```python
from build123d import *

# Parameters (mm, degrees)
SKETCH1_W           = 200
SKETCH1_H           = 200
BOSS_EXTRUDE1_DEPTH = 300
FILLET1_R           = 10
SHELL1_T            = -8
CUT_EXTRUDE1_DEPTH  = 44
FILLET2_R           = 25
FILLET3_R           = 25
CUT_EXTRUDE2_DEPTH  = 5.5


with BuildPart() as part:
    # Sketch1 → Boss-Extrude1 (new body)
    with BuildSketch(Plane(origin=(0, 0, 0), x_dir=(1, 0, 0), z_dir=(0, 1, 0))):
        Rectangle(SKETCH1_W, SKETCH1_H)
    extrude(amount=BOSS_EXTRUDE1_DEPTH)

    # Fillet1
    fillet1_edges = [part.edges().sort_by_distance(p)[0] for p in [
        (0, 0, -100),
        (100, 0, 0),
        (0, 0, 100),
        (-100, 0, 0),
        (-100, 150, -100),
        (100, 150, -100),
        (100, 150, 100),
        (-100, 150, 100),
    ]]
    fillet(fillet1_edges, radius=FILLET1_R)

    # Shell1
    shell1_openings = [part.faces().sort_by_distance(p)[0] for p in [
        (0, 300, 0),
    ]]
    offset(amount=SHELL1_T, openings=shell1_openings, kind=Kind.INTERSECTION)

    # Sketch2 → Cut-Extrude1 (cut)
    with BuildSketch(Plane(origin=(0, 0, -100), x_dir=(-1, 0, 0), z_dir=(0, 0, -1))):
        with BuildLine():
            Line((62, 100), (-28, 100))
            Line((-28, 100), (-28, 130))
            ThreePointArc((-28, 130), (-57.029416855, 206), (-28, 282))
            Line((-28, 282), (-28, 300))
            Line((-28, 300), (62, 300))
            Line((62, 300), (62, 100))
        make_face()
    extrude(amount=-CUT_EXTRUDE1_DEPTH, mode=Mode.SUBTRACT)

    # Fillet2
    fillet2_edges = [part.edges().sort_by_distance(p)[0] for p in [
        (28, 130, -96),
    ]]
    fillet(fillet2_edges, radius=FILLET2_R)

    # Fillet3
    fillet3_edges = [part.edges().sort_by_distance(p)[0] for p in [
        (28, 282, -96),
    ]]
    fillet(fillet3_edges, radius=FILLET3_R)

    # Sketch3 → Cut-Extrude2 (cut)
    with BuildSketch(Plane(origin=(0, 300, 0), x_dir=(1, 0, 0), z_dir=(0, 1, 0))):
        with BuildLine():
            Line((28, 92), (90, 92))
            ThreePointArc((90, 92), (91.414213562, 91.414213562), (92, 90))
            Line((92, 90), (92, -90))
            ThreePointArc((92, -90), (91.414213562, -91.414213562), (90, -92))
            Line((90, -92), (-90, -92))
            ThreePointArc((-90, -92), (-91.414213562, -91.414213562), (-92, -90))
            Line((-92, -90), (-92, 90))
            ThreePointArc((-92, 90), (-91.414213562, 91.414213562), (-90, 92))
            Line((-90, 92), (-62, 92))
            Line((-62, 92), (-62, 94.5))
            Line((-62, 94.5), (-90, 94.5))
            ThreePointArc((-90, 94.5), (-93.181980515, 93.181980515), (-94.5, 90))
            Line((-94.5, 90), (-94.5, -90))
            ThreePointArc((-94.5, -90), (-93.181980515, -93.181980515), (-90, -94.5))
            Line((-90, -94.5), (90, -94.5))
            ThreePointArc((90, -94.5), (93.181980515, -93.181980515), (94.5, -90))
            Line((94.5, -90), (94.5, 90))
            ThreePointArc((94.5, 90), (93.181980515, 93.181980515), (90, 94.5))
            Line((90, 94.5), (28, 94.5))
            Line((28, 94.5), (28, 92))
        make_face()
    extrude(amount=-CUT_EXTRUDE2_DEPTH, mode=Mode.SUBTRACT)


solid = part.part
```
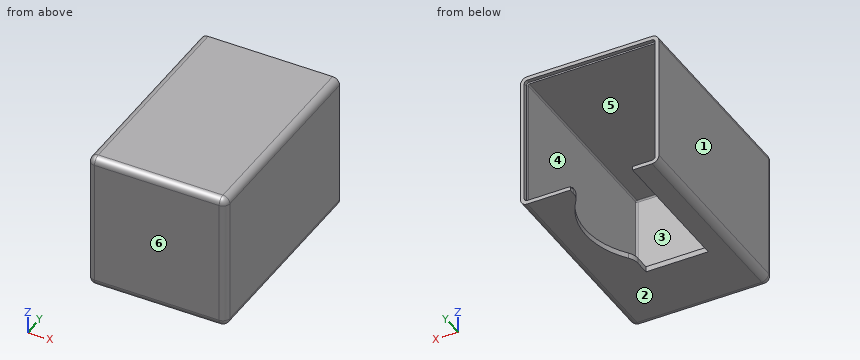
Geometry: final body of the model. Coordinates: model frame, mm. Face numbers are marked on the shaded views. A direction names the side the tool comes from. Coordinates: 2 decimals unless noted, no trailing zeros. Order: outer loops, then holes, each group sorted by start corner. A loop starts at its lowest first (then second) coordinate and runs counter-clockwise, first axis right, second up. Notation, with made-up numbers: (67, -1.5) - (110, -1.5) arc R19 ccw to (110, 22.5) - close; hole circle Ø10 at (-12, -36). An arc over 180 degrees is marked (long way). Return JSON: item names as keys, results as strings. Group by question number.
1. Cut plane B-B (x = -84). Output: boundary loops of the cut face in (y, z).
2. Pin query (flat end, axial travel): pin 1 (4 mm diameter, centred on y = 108.5, z = -94.5, fed in from -X); pin 2 (6 mm diameter, centred on x = -50.5, z = 62.5, fed in from +Y); pin 3 (4 mm diameter, centred on y = 295.5, z = -97, fed in from -X). Return the tip coordinate at first contact, or that it passes through.
3. Cut plane C-C (y = 71). Output: boundary loops of the cut face in (x, z).
4. Cut plane D-D (z = 46). Output: boundary loops of the cut face in (x, y).
5. Cut plane A-A (y = 104). Output: boundary loops of the cut face in (x, z), plus the area to 3 significant figures.
6. Set-up query: the marked faces 5 and 6. Return all of +Z, -Z, +X, -X, +Y, -Y with unobstructed straight access to the full face (end or side cutting, diameter ignored); none if empty.
7. Material intervals for line 1 along Z through (x, y) = (65.5, 110.5); line 2 along Y through (x, z) = (47, 18), sorted ascending. Write a range as [from, to].
8. Pull-direction query (X, two-part tool) for the marked faces 1, 2, 3 and 4; classes: pulls with the +X half, pulls with the -X half, needs draft (parallel to the pull), parting line crosses it, or undercut.
Resolved:
{
 "1": {"outline": "(0, -90) arc R10 ccw to (10, -100) - (300, -100) - (300, -94.5) - (294.5, -94.5) - (294.5, -92) - (10, -92) arc R2 cw to (8, -90) - (8, 90) arc R2 cw to (10, 92) - (294.5, 92) - (294.5, 94.5) - (300, 94.5) - (300, 100) - (10, 100) arc R10 ccw to (0, 90) - close"},
 "2": {"pin 1": "stops at x = -99.68", "pin 2": "stops at y = 8", "pin 3": "stops at x = -98.66"},
 "3": {"outline": "(-100, -90) arc R10 ccw to (-90, -100) - (90, -100) arc R10 ccw to (100, -90) - (100, 90) arc R10 ccw to (90, 100) - (-90, 100) arc R10 ccw to (-100, 90) - close; hole (-92, -90) arc R2 ccw to (-90, -92) - (90, -92) arc R2 ccw to (92, -90) - (92, 90) arc R2 ccw to (90, 92) - (-90, 92) arc R2 ccw to (-92, 90) - close"},
 "4": {"outline": "(-100, 10) arc R10 ccw to (-90, 0) - (90, 0) arc R10 ccw to (100, 10) - (100, 300) - (94.5, 300) - (94.5, 294.5) - (92, 294.5) - (92, 10) arc R2 cw to (90, 8) - (-90, 8) arc R2 cw to (-92, 10) - (-92, 294.5) - (-94.5, 294.5) - (-94.5, 300) - (-100, 300) - close"},
 "5": {"outline": "(-100, -90) arc R10 ccw to (-90, -100) - (-62, -100) - (-62, -92) - (-90, -92) arc R2 cw to (-92, -90) - (-92, 90) arc R2 cw to (-90, 92) - (90, 92) arc R2 cw to (92, 90) - (92, -90) arc R2 cw to (90, -92) - (28, -92) - (28, -100) - (90, -100) arc R10 ccw to (100, -90) - (100, 90) arc R10 ccw to (90, 100) - (-90, 100) arc R10 ccw to (-100, 90) - close", "area": "5,340 mm²"},
 "6": {"face 5": "+Y", "face 6": "+Z, -Z, +X, -X, -Y"},
 "7": {"line 1": "z = [-100, -92], [92, 100]", "line 2": "y = [0, 8]"},
 "8": {"face 1": "pulls with the -X half", "face 2": "needs draft", "face 3": "undercut", "face 4": "undercut"}
}
